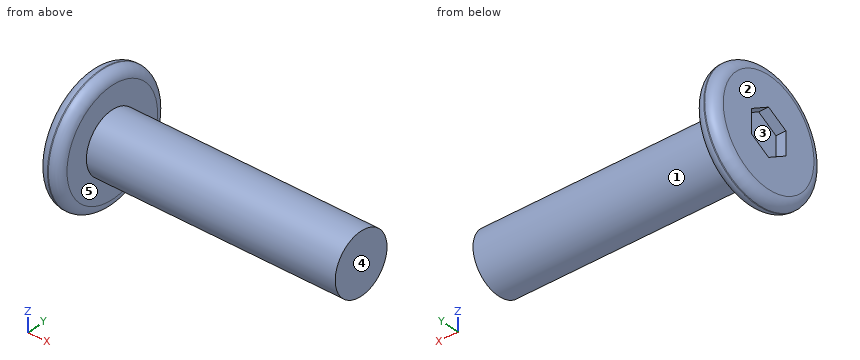
```python
from build123d import *

# Parameters (mm, degrees)
FILLET_1_R          = 1
CUT_EXTRUDE_1_DEPTH = 1


with BuildPart() as part:
    # 草图1 → 旋转1 (revolve)
    with BuildSketch(Plane.XY):
        Polygon((0, 0), (0, 6.25), (2.1, 6.25), (2.1, 3), (27.1, 3), (27.1, 0), align=None)
    revolve(axis=Axis((27.1, 0, 0), (-1, 0, 0)))

    # 圆角1
    fillet_1_edges = [part.edges().sort_by_distance(p)[0] for p in [
        (2.1, -6.25, 0),
        (0, -6.25, 0),
    ]]
    fillet(fillet_1_edges, radius=FILLET_1_R)

    # 草图2 → 切除-拉伸1 (cut)
    with BuildSketch(Plane.ZY):
        Polygon((1.154700538, 2), (-1.154700538, 2), (-2.309401077, 0), (-1.154700538, -2), (1.154700538, -2), (2.309401077, 0), align=None)
    extrude(amount=-CUT_EXTRUDE_1_DEPTH, mode=Mode.SUBTRACT)


solid = part.part
```
Verification items for the finished model (mm, model axes). Face numbers are marked on the shaded views. A direction names the side the tool comes from. Give positions to 0.01 mm unless a question says otherwise; leave off trailing zeros. Order: outer loops, then holes, each group sorted by start corner. A loop starts at its lowest first (then second) coordinate and runs counter-clockwise, first axis right, second up. Notation, with made-up numbers: (17, 9) -> (66, 9) arc R16 cw to (66, 39) -> close; hole circle Ø10 at (44.5, 60). An arc over 180 degrees is marked (long way). Use a Markdown table: item, result.
1) Section check B-B, the plane x = 14. Record the boundary of the cut face in (y, z), then the cut area to 3 significant figures.
Results:
| item | result |
|---|---|
| outline | circle Ø6 at (0, 0) |
| area | 28.3 mm² |
2) Depth check by flat-ended pin: pin 1 Ø5 at (x, y) = (7.5, 1.5) entering from -Z; pin 2 Ø0.8 at (x, z) = (0.5, -0.5) entering from +Y; pin 3 Ø6 at (x, y) = (15.5, -0.5) entering from +Z; pin 4 Ø2 at (x, y) = (7, -4.5) entering from -Z (3 decimals). Enter the tip coordinate at first touch or a pass-through.
Results:
| item | result |
|---|---|
| pin 1 | z = -3 |
| pin 2 | y = 6.23 |
| pin 3 | z = 3 |
| pin 4 | through |
3) Section check A-A, the plane z = 0. Record the boundary of the cut face in (x, y).
Results:
| item | result |
|---|---|
| outline | (0, -5.25) arc R1 ccw to (1, -6.25) -> (1.1, -6.25) arc R1 ccw to (2.1, -5.25) -> (2.1, -3) -> (27.1, -3) -> (27.1, 3) -> (2.1, 3) -> (2.1, 5.25) arc R1 ccw to (1.1, 6.25) -> (1, 6.25) arc R1 ccw to (0, 5.25) -> (0, 2) -> (1, 2) -> (1, -2) -> (0, -2) -> close |
4) Tool access check on the marked faces 4 and 5. Record the directions out of +Z, -Z, +X, -X, +Y, -Y that give a thin tool (end or side, any length) a straight path to the whole face; none if there is none.
Results:
| item | result |
|---|---|
| face 4 | +Z, -Z, +X, +Y, -Y |
| face 5 | +X |
5) Material ranges on probe 1 along X at (y, z) = (-3.25, 3.25); probe 2 along Y at (x, z) = (15.5, -0.25); probe 3 along Y at (x, z) = (13.5, -2), recorded low to high.
Results:
| item | result |
|---|---|
| probe 1 | 0 to 2.1 |
| probe 2 | -2.99 to 2.99 |
| probe 3 | -2.24 to 2.24 |
6) Mould release check, pull along Y, two halves, no side actions. Record for the marked faces 1, 2 and 3: pulls with the +Y half, pulls with the -Y half, needs draft (parallel to the pull), parting line crosses it, or undercut.
Results:
| item | result |
|---|---|
| face 1 | parting line crosses it |
| face 2 | needs draft |
| face 3 | undercut |
